For this review, take the finished solid that the model builds, in its own axes (mm). A direction names the side the tool comes from. Coordinates: 2 decimals unless noted, no trailing zeros. Loops run counter-clockwise (first coordinate to the right, second up) from the corner with the lowest first, then second, coordinate; pieces in that order, holes last.
1. Take a section at A-A, the plane x = 60. Count the separate pieces of the cut face and the enclosed holes in it, then the cut area to 3 significant figures.
2. Machinability: for faces 1 (the face through (62, 8, 5)), 2 (the face through (97, 2, 2)), which of the approach directions +Z, -Z, +X, -X, +Y, -Y give a long, thin tool a straight path to every point of the face, cutting with its end or side? Answer none if there is none.
3. To check wall thickness, follow probe 1 along Y at (x, z) = (10, 2.25); probe 2 along Y at (x, z) = (61, 0.75). State the ranges of each line that lie inside material, in increasing order.
4. Take a section at C-C, the plane y = 10. State the section outline as (x, z) points.
5. Clearance check with flat-ended pins moving along their axes: P1, Ø6, axis at x = 47.5, y = 69.5, coming from the -Z side; P2, Ø2.5, axis at x = 61.5, y = 31, coming from the +Z side; P3, Ø7, axis at x = 58, y = 10.5, coming from the +Z side; P4, Ø4, axis at x = 44, z = 5.5, coming from the +Y side. State where each tip first meets the part, or that it passes through.
6. Mouldability with a two-part tool opening along X and no side actions: class faces 3 (the face through (3.1, 96.5, 6.6)), 4 (the face through (96.5, 3.1, 6.6)), 5 (the face through (64.16, 28.28, 7.54)) as pulls with the +X half, pulls with the -X half, needs draft (parallel to the pull), parting line crosses it, or undercut.
7. Take a section at B-B, the plane z = 2.25. State the section outline as (x, y) points, then the cut area to 3 significant figures.
```python
from build123d import *

# Parameters (mm, degrees)
BOSS_EXTRUDE1_DEPTH     = 10
SKETCH2_R               = 2.6
CUT_EXTRUDE1_DEPTH      = 142.774468788
SKETCH3_W               = 60
SKETCH3_H               = 9
SKETCH3_W_2             = 9
SKETCH3_H_2             = 60
BOSS_EXTRUDE3_DEPTH     = 1.46
CUT_EXTRUDE2_DEPTH      = 142.774468788
CUT_EXTRUDE2_DEPTH_BACK = 142.774468788
SKETCH2_2_R             = 2.6
CHAMFER1_SIZE           = 1.46
CUT_EXTRUDE3_START      = 10
SKETCH4_R               = 4.5
CUT_EXTRUDE3_DEPTH      = 5
CHAMFER2_SIZE           = 5


with BuildPart() as part:
    # Sketch1 → Boss-Extrude1 (new body)
    with BuildSketch(Plane.XY):
        Polygon((0, 0), (100, 0), (100, 40), (20, 100), (0, 100), align=None)
    extrude(amount=BOSS_EXTRUDE1_DEPTH)

    # Sketch2 → Cut-Extrude1 (cut, through all)
    with BuildSketch(Plane.XY):
        with Locations((10, 85)):
            Circle(SKETCH2_R)
        with Locations((10, 60)):
            Circle(SKETCH2_R)
        with Locations((85, 30)):
            Circle(SKETCH2_R)
        with Locations((85, 10)):
            Circle(SKETCH2_R)
        with Locations((60, 10)):
            Circle(SKETCH2_R)
        with Locations((60, 30)):
            Circle(SKETCH2_R)
    extrude(amount=CUT_EXTRUDE1_DEPTH, mode=Mode.SUBTRACT)

    # Sketch3 → Boss-Extrude3 (add)
    with BuildSketch(Plane.XY):
        with Locations((70, 30)):
            Rectangle(SKETCH3_W, SKETCH3_H)
        with Locations((70, 10)):
            Rectangle(SKETCH3_W, SKETCH3_H)
        with Locations((10, 70)):
            Rectangle(SKETCH3_W_2, SKETCH3_H_2)
    extrude(amount=-BOSS_EXTRUDE3_DEPTH)

    # Sketch2<2> → Cut-Extrude2 (cut, two sides: drawn at the far end of the back side and taken through both)
    with BuildSketch(Plane.XY.offset(-CUT_EXTRUDE2_DEPTH_BACK)):
        with Locations((10, 85)):
            Circle(SKETCH2_2_R)
        with Locations((10, 60)):
            Circle(SKETCH2_2_R)
        with Locations((85, 30)):
            Circle(SKETCH2_2_R)
        with Locations((85, 10)):
            Circle(SKETCH2_2_R)
        with Locations((60, 10)):
            Circle(SKETCH2_2_R)
        with Locations((60, 30)):
            Circle(SKETCH2_2_R)
    extrude(amount=CUT_EXTRUDE2_DEPTH + CUT_EXTRUDE2_DEPTH_BACK, mode=Mode.SUBTRACT)

    # Chamfer1
    chamfer1_edges = [part.edges().sort_by_distance(p)[0] for p in [
        (14.5, 70, -1.46),
        (5.5, 70, -1.46),
        (70, 5.5, -1.46),
        (70, 14.5, -1.46),
        (70, 25.5, -1.46),
        (70, 34.5, -1.46),
    ]]
    chamfer(chamfer1_edges, length=CHAMFER1_SIZE - 0.0001)  # a hair under: the kernel refuses the full size

    # Sketch4 → Cut-Extrude3 (cut)
    with BuildSketch(Plane.XY.offset(CUT_EXTRUDE3_START)):
        with Locations((10, 85)):
            Circle(SKETCH4_R)
        with Locations((10, 60)):
            Circle(SKETCH4_R)
        with Locations((60, 30)):
            Circle(SKETCH4_R)
        with Locations((85, 30)):
            Circle(SKETCH4_R)
        with Locations((85, 10)):
            Circle(SKETCH4_R)
        with Locations((60, 10)):
            Circle(SKETCH4_R)
    extrude(amount=-CUT_EXTRUDE3_DEPTH, mode=Mode.SUBTRACT)

    # Chamfer2
    chamfer2_edges = [part.edges().sort_by_distance(p)[0] for p in [
        (100, 20, 10),
        (60, 70, 10),
        (10, 100, 10),
        (0, 50, 10),
        (50, 0, 10),
        (0, 100, 5),
        (100, 0, 5),
        (0, 0, 5),
    ]]
    chamfer(chamfer2_edges, length=CHAMFER2_SIZE)


solid = part.part
```
Results list:
1. separate pieces: 3
1. enclosed holes: 0
1. area: 537 mm2
2. face 1: +Z
2. face 2: +Z, -Z, +X, -Y
3. probe 1: y = 0 to 57.4, 62.6 to 82.4, 87.6 to 100
3. probe 2: y = 0 to 7.6, 12.4 to 27.6, 32.4 to 69.25
4. outline: (0, 0) - (40, 0) - (40, -1.46) - (57.4, -1.46) - (57.4, 5) - (55.5, 5) - (55.5, 10) - (5, 10) - (0, 5) - close; (62.6, -1.46) - (82.4, -1.46) - (82.4, 5) - (80.5, 5) - (80.5, 10) - (64.5, 10) - (64.5, 5) - (62.6, 5) - close; (87.6, -1.46) - (100, -1.46) - (100, 5) - (95, 10) - (89.5, 10) - (89.5, 5) - (87.6, 5) - close
5. P1: stops at z = 0
5. P2: stops at z = 5
5. P3: stops at z = 10
5. P4: stops at y = 83.45
6. face 3: pulls with the -X half
6. face 4: pulls with the +X half
6. face 5: undercut
7. outline: (0, 5) - (5, 0) - (95, 0) - (100, 5) - (100, 40) - (20, 100) - (5, 100) - (0, 95) - close; hole circle Ø5.2 at (10, 60); hole circle Ø5.2 at (10, 85); hole circle Ø5.2 at (60, 10); hole circle Ø5.2 at (60, 30); hole circle Ø5.2 at (85, 10); hole circle Ø5.2 at (85, 30)
7. area: 7,440 mm2
